from build123d import *

# Parameters (mm, degrees)
SKETCH_1_W           = 94
SKETCH_1_H           = 26
SKETCH_1_R           = 1
EXTRUDE_1_DEPTH      = 3.5
SKETCH_2_W           = 4.7
SKETCH_2_H           = 8.9
SKETCH_2_W_2         = 59.6
SKETCH_2_H_2         = 6.6
CUT_EXTRUDE_1_DEPTH  = 49.890183064
SKETCH_3_R           = 1.5
CUT_EXTRUDE_2_DEPTH  = 49.890183064
SKETCH_4_R           = 1.75
CUT_EXTRUDE_3_DEPTH  = 2
SKETCH_5_W           = 7.8
SKETCH_5_H           = 2.6
SKETCH_5_W_2         = 8.6
SKETCH_5_H_2         = 2
CUT_EXTRUDE_4_DEPTH  = 6
SKETCH_5_3_W         = 15.6
SKETCH_5_3_H         = 2
CUT_EXTRUDE_5_DEPTH  = 20
SKETCH_6_W           = 70
SKETCH_6_H           = 19.6
SKETCH_6_W_2         = 18.8
SKETCH_6_H_2         = 3
SKETCH_6_W_3         = 82.8
SKETCH_6_H_3         = 11
SKETCH_6_W_4         = 3.2
SKETCH_6_H_4         = 5.2
CUT_EXTRUDE_12_DEPTH = 2
SKETCH_7_W           = 6.7
SKETCH_7_H           = 7.7
CUT_EXTRUDE_13_DEPTH = 0.5
SKETCH_8_W           = 7.4
SKETCH_8_H           = 0.9
SKETCH_8_W_2         = 15.6
SKETCH_8_H_2         = 1.5
EXTRUDE_2_DEPTH      = 2.1
SKETCH_10_W          = 19.8
SKETCH_10_H          = 1.9
SKETCH_10_W_2        = 11.8
SKETCH_10_H_2        = 4.2
EXTRUDE_3_DEPTH      = 2


with BuildPart() as part:
    # 草图1 → 凸台-拉伸1 (new body)
    with BuildSketch(Plane(origin=(0, 0, 0), x_dir=(1, 0, 0), z_dir=(0, 1, 0))):
        Rectangle(SKETCH_1_W, SKETCH_1_H)
        with Locations(Location((-44, 10, 0), (0, 0, 270))):
            Circle(SKETCH_1_R, mode=Mode.SUBTRACT)
        with Locations(Location((-44, -10, 0), (0, 0, 270))):
            Circle(SKETCH_1_R, mode=Mode.SUBTRACT)
        with Locations(Location((44, 10, 0), (0, 0, 270))):
            Circle(SKETCH_1_R, mode=Mode.SUBTRACT)
        with Locations(Location((44, -10, 0), (0, 0, 270))):
            Circle(SKETCH_1_R, mode=Mode.SUBTRACT)
    extrude(amount=EXTRUDE_1_DEPTH)

    # 草图2 → 切除-拉伸1 (cut, through all)
    with BuildSketch(Plane.XZ):
        with Locations((-44.65, 2.65)):
            Rectangle(SKETCH_2_W, SKETCH_2_H)
        with Locations((-4.8, 0)):
            Rectangle(SKETCH_2_W_2, SKETCH_2_H_2)
    extrude(amount=-CUT_EXTRUDE_1_DEPTH, mode=Mode.SUBTRACT)

    # 草图3 → 切除-拉伸2 (cut, through all)
    with BuildSketch(Plane(origin=(0, 0, 0), x_dir=(-1, 0, 0), z_dir=(0, -1, 0))):
        with Locations(Location((27.5, -10, 0), (0, 0, 90))):
            Circle(SKETCH_3_R)
    extrude(amount=-CUT_EXTRUDE_2_DEPTH, mode=Mode.SUBTRACT)

    # 草图4 → 切除-拉伸3 (cut)
    with BuildSketch(Plane.XZ):
        with Locations(Location((-44, 10, 0), (0, 0, 270))):
            Circle(SKETCH_4_R)
        with Locations(Location((-44, -10, 0), (0, 0, 270))):
            Circle(SKETCH_4_R)
        with Locations(Location((44, 10, 0), (0, 0, 270))):
            Circle(SKETCH_4_R)
        with Locations(Location((44, -10, 0), (0, 0, 270))):
            Circle(SKETCH_4_R)
    extrude(amount=-CUT_EXTRUDE_3_DEPTH, mode=Mode.SUBTRACT)

    # 草图5 → 切除-拉伸4 (cut)
    with BuildSketch(Plane.XY.offset(13)):
        with Locations((-37.2, 2.2)):
            Rectangle(SKETCH_5_W, SKETCH_5_H)
        with Locations((-27.5, 2.5)):
            Rectangle(SKETCH_5_W_2, SKETCH_5_H_2)
    extrude(amount=-CUT_EXTRUDE_4_DEPTH, mode=Mode.SUBTRACT)

    # 草图5<3> → 切除-拉伸5 (cut)
    with BuildSketch(Plane.XY.offset(13)):
        with Locations((32.9, 2.5)):
            Rectangle(SKETCH_5_3_W, SKETCH_5_3_H)
    extrude(amount=-CUT_EXTRUDE_5_DEPTH, mode=Mode.SUBTRACT)

    # 草图6 → 切除-拉伸12 (cut)
    with BuildSketch(Plane(origin=(0, 3.5, 0), x_dir=(1, 0, 0), z_dir=(0, 1, 0))):
        with Locations((-7.8, 2.7)):
            Rectangle(SKETCH_6_W, SKETCH_6_H)
        with Locations((36.6, 0)):
            Rectangle(SKETCH_6_W_2, SKETCH_6_H_2)
        with Locations((0.3, -7)):
            Rectangle(SKETCH_6_W_3, SKETCH_6_H_3)
        with Locations((-44.4, 5.4)):
            Rectangle(SKETCH_6_W_4, SKETCH_6_H_4)
    extrude(amount=-CUT_EXTRUDE_12_DEPTH, mode=Mode.SUBTRACT)

    # 草图7 → 切除-拉伸13 (cut)
    with BuildSketch(Plane(origin=(0, 1.5, 0), x_dir=(1, 0, 0), z_dir=(0, 1, 0))):
        with Locations((-27.35, 7.15)):
            Rectangle(SKETCH_7_W, SKETCH_7_H)
    extrude(amount=-CUT_EXTRUDE_13_DEPTH, mode=Mode.SUBTRACT)

    # 草图8 → 凸台-拉伸2 (add)
    with BuildSketch(Plane.XY.offset(13)):
        with Locations((-37.2, 0.45)):
            Rectangle(SKETCH_8_W, SKETCH_8_H)
        with Locations((32.9, 0.75)):
            Rectangle(SKETCH_8_W_2, SKETCH_8_H_2)
    extrude(amount=EXTRUDE_2_DEPTH)

    # 草图10 → 凸台-拉伸3 (add)
    with BuildSketch(Plane.ZY.offset(47)):
        with Locations((0, 0.95)):
            Rectangle(SKETCH_10_W, SKETCH_10_H)
        with Locations((0, 2.1)):
            Rectangle(SKETCH_10_W_2, SKETCH_10_H_2)
    extrude(amount=EXTRUDE_3_DEPTH)


solid = part.part
Design review of the part built by this model. Coordinates are the model's own, in mm. A direction names the side the tool comes from. Round coordinates to 2 decimals unless told otherwise and drop trailing zeros. Loops run counter-clockwise (first coordinate to the right, second up) from the corner with the lowest first, then second, coordinate; pieces in that order, holes last. Notation, with made-up numbers: (80, 26) -> (104, 26) arc R15 ccw to (104, 39) -> close; hole circle Ø7 at (16.25, 34.25). An arc over 180 degrees is marked (long way). Use one line per item in the form item = value. Start each with the question number.
Q1. Machinability: for faces 4 (the face through (44, 3, 1.5)), 5 (the face through (-45.71, 0.99, -9.62)), 6 (the face through (-48, 1.9, -8)), 7 (the face through (-37, 0.9, 11)), which of the approach directions +Z, -Z, +X, -X, +Y, -Y give a long, thin tool a straight path to every point of the face, cutting with its end or side? Answer none if there is none.
Q2. We need section B-B on x = 44. Give the boundary of the cut face in (y, z).
Q3. We need section D-D on x = -27.5. Give the boundary of the cut face in (y, z).
Q4. For pin 1 Ø1.6 at (x, y) = (-48, 3.5) entering from -Z; pin 2 Ø1.8 at (x, z) = (44, 10) entering from -Y (3 decimals); pin 3 Ø6 at (x, z) = (-39, 12) entering from +Y; pin 4 Ø0.6 at (y, z) = (3, 7.5) entering from -X, all flat-tipped, find the tip position at first contact; note any pin that passes through.
Q5. We need section A-A on x = -44. Give the boundary of the cut face in (y, z), then the cut area to 4 significant figures.
Q6. Wall thickness on line 1 along X through (y, z) = (2.4, -10); line 2 along Z through (x, y) = (44, 2.7); line 3 along X through (y, z) = (2.8, -4): over which ranges is each line inside the solid? List them lowest first. Write a range as [from, to].
Q7. Draft analysis for pull direction Z (two halves, no side actions). For faces 1 (the face through (-48, 1.9, 8)), 2 (the face through (-44, 3, -8)), 3 (the face through (-1, 2, -13)), state which applies: +Z half, -Z half, draft (parallel to the pull), parting line (faces both ways), or undercut.
Q8. We need section C-C on x = -6. Give the boundary of the cut face in (y, z).
Calculated:
q1.face_4 = +Y
q1.face_5 = -Y
q1.face_6 = -Z, -X, +Y
q1.face_7 = +Z, +Y
q2.outline = (0, -13) -> (3.5, -13) -> (3.5, -11) -> (2, -11) -> (2, -11.75) -> (0, -11.75) -> close; (0, -8.25) -> (2, -8.25) -> (2, -9) -> (3.5, -9) -> (3.5, -1.5) -> (1.5, -1.5) -> (1.5, 1.5) -> (3.5, 1.5) -> (3.5, 9) -> (2, 9) -> (2, 8.25) -> (0, 8.25) -> close; (0, 11.75) -> (2, 11.75) -> (2, 11) -> (3.5, 11) -> (3.5, 13) -> (0, 13) -> close
q3.outline = (0, -13) -> (3.5, -13) -> (3.5, -12.5) -> (1.5, -12.5) -> (1.5, -11) -> (1, -11) -> (1, -3.3) -> (0, -3.3) -> close; (0, 3.3) -> (1.5, 3.3) -> (1.5, 8.5) -> (0, 8.5) -> close; (0, 11.5) -> (1.5, 11.5) -> (1.5, 13) -> (0, 13) -> close
q4.pin_1 = -5.9
q4.pin_2 = through
q4.pin_3 = 3.5
q4.pin_4 = -47
q5.outline = (0, -13) -> (3.5, -13) -> (3.5, -11) -> (2, -11) -> (2, -11.75) -> (0, -11.75) -> close; (0, -8.25) -> (2, -8.25) -> (2, -9) -> (3.5, -9) -> (3.5, -8) -> (1.5, -8) -> (1.5, -2.8) -> (3.5, -2.8) -> (3.5, -1.8) -> (0, -1.8) -> close; (0, 7.1) -> (3.5, 7.1) -> (3.5, 9) -> (2, 9) -> (2, 8.25) -> (0, 8.25) -> close; (0, 11.75) -> (2, 11.75) -> (2, 11) -> (3.5, 11) -> (3.5, 13) -> (0, 13) -> close
q5.area = 29.45 mm²
q6.line_1 = [-47, -45], [-43, -42.8], [27.2, 43], [45, 47]
q6.line_2 = [-13, -11], [-9, -1.5], [1.5, 9], [11, 13]
q6.line_3 = [-49, -46], [40.7, 47]
q7.face_1 = draft
q7.face_2 = undercut
q7.face_3 = -Z half
q8.outline = (0, -13) -> (3.5, -13) -> (3.5, -12.5) -> (1.5, -12.5) -> (1.5, -3.3) -> (0, -3.3) -> close; (0, 3.3) -> (1.5, 3.3) -> (1.5, 12.5) -> (3.5, 12.5) -> (3.5, 13) -> (0, 13) -> close
